```python
from build123d import *

# Parameters (mm, degrees)
SKETCH1_R           = 60
SKETCH1_R_2         = 20
BOSS_EXTRUDE1_DEPTH = 15
SKETCH2_R           = 7.5
CUT_EXTRUDE1_DEPTH  = 15


with BuildPart() as part:
    # Sketch1 → Boss-Extrude1 (new body)
    with BuildSketch(Plane.XY):
        Circle(SKETCH1_R)
        Circle(SKETCH1_R_2, mode=Mode.SUBTRACT)
    extrude(amount=BOSS_EXTRUDE1_DEPTH)

    # Sketch2 → Cut-Extrude1 (cut)
    with BuildSketch(Plane.XY.offset(15)):
        with Locations((0, 60)):
            Circle(SKETCH2_R)
        with Locations((18.541019662, 57.063390978)):
            Circle(SKETCH2_R)
        with Locations((35.267115138, 48.541019663)):
            Circle(SKETCH2_R)
        with Locations((48.541019663, 35.267115138)):
            Circle(SKETCH2_R)
        with Locations((57.063390978, 18.541019663)):
            Circle(SKETCH2_R)
        with Locations((60, 0)):
            Circle(SKETCH2_R)
        with Locations((57.063390978, -18.541019662)):
            Circle(SKETCH2_R)
        with Locations((48.541019663, -35.267115138)):
            Circle(SKETCH2_R)
        with Locations((35.267115138, -48.541019662)):
            Circle(SKETCH2_R)
        with Locations((18.541019663, -57.063390978)):
            Circle(SKETCH2_R)
        with Locations((0, -60)):
            Circle(SKETCH2_R)
        with Locations((-18.541019662, -57.063390978)):
            Circle(SKETCH2_R)
        with Locations((-35.267115138, -48.541019663)):
            Circle(SKETCH2_R)
        with Locations((-48.541019662, -35.267115138)):
            Circle(SKETCH2_R)
        with Locations((-57.063390978, -18.541019663)):
            Circle(SKETCH2_R)
        with Locations((-60, 0)):
            Circle(SKETCH2_R)
        with Locations((-57.063390978, 18.541019662)):
            Circle(SKETCH2_R)
        with Locations((-48.541019662, 35.267115138)):
            Circle(SKETCH2_R)
        with Locations((-35.267115138, 48.541019662)):
            Circle(SKETCH2_R)
        with Locations((-18.541019662, 57.063390978)):
            Circle(SKETCH2_R)
    extrude(amount=-CUT_EXTRUDE1_DEPTH, mode=Mode.SUBTRACT)


solid = part.part
```
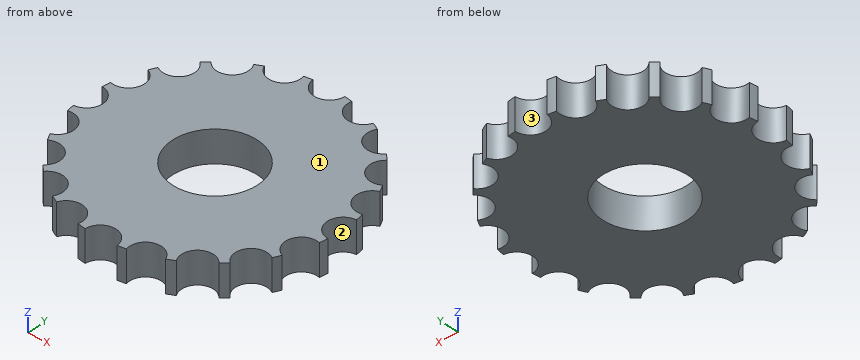
Can you work these out from the model? Positions are in its coordinate system, mm. Face numbers are marked on the shaded views. Give positions to 0.01 mm unless a question says otherwise; leave off trailing zeros. Order: outer loops, then holes, each group sorted by start corner. A loop starts at its lowest first (then second) coordinate and runs counter-clockwise, first axis right, second up. Notation, with made-up numbers: (-28, 34.25) - (4, 34.25) arc R23 cw to (4, 57.25) - close; hole circle Ø4 at (87.25, 13.5). An arc over 180 degrees is marked (long way). Use a Markdown table: item, result. Add a question column.
Q1. I'm going to push flat-ended pins straight in: pin 1 (2 mm diameter, centred on y = 5, z = 11.5, fed in from +X); pin 2 (3 mm diameter, centred on y = 29.5, z = 7, fed in from -X); pin 3 (5 mm diameter, centred on y = 44.5, z = 12, fed in from -X). Where does each tip first touch, or does it pass through?
Q2. If we section it at D-D on y = -39.5: Write out the boundary of the cut face in (x, z), plus the area to 3 significant figures.
Q3. Please list where these lines run through material, in increasing order: line 1 along Y through (x, z) = (0, 4); line 2 along Y through (x, z) = (-1, 3.5); line 3 along Y through (x, z) = (-51, 4.25).
Q4. If we section it at A-A on y = 0: Write out the boundary of the cut face in (x, z), plus the area to 3 significant figures.
Q5. If we section it at B-B on x = -5.5: Write out the boundary of the cut face in (y, z).
Q6. If we section it at C-C on y = 35: Write out the boundary of the cut face in (x, z), plus the area to 3 significant figures.
Q7. If we mould it in two halves opening along X, with no side actions, what happens to the marked faces 1, 2 and 3? For each: released by +X, released by -X, zero draft, split by the parting line, or undercut.
Answers follow:
| question | item | result |
|---|---|---|
| 1 | pin 1 | stops at x = 55.5 |
| 1 | pin 2 | stops at x = -53.07 |
| 1 | pin 3 | stops at x = -42.85 |
| 2 | outline | (-42.35, 0) - (42.35, 0) - (42.35, 15) - (-42.35, 15) - close |
| 2 | area | 1,270 mm^2 |
| 3 | line 1 | y = -52.5 to -20, 20 to 52.5 |
| 3 | line 2 | y = -52.57 to -19.97, 19.97 to 52.57 |
| 3 | line 3 | y = -28.18 to -22.96, -14.13 to 14.13, 22.96 to 28.18 |
| 4 | outline | (-52.5, 0) - (-20, 0) - (-20, 15) - (-52.5, 15) - close; (20, 0) - (52.5, 0) - (52.5, 15) - (20, 15) - close |
| 4 | area | 975 mm^2 |
| 5 | outline | (-54.9, 0) - (-19.23, 0) - (-19.23, 15) - (-54.9, 15) - close; (19.23, 0) - (54.9, 0) - (54.9, 15) - (19.23, 15) - close |
| 6 | outline | (-41.05, 0) - (41.05, 0) - (41.05, 15) - (-41.05, 15) - close |
| 6 | area | 1,230 mm^2 |
| 7 | face 1 | zero draft |
| 7 | face 2 | released by +X |
| 7 | face 3 | undercut |
